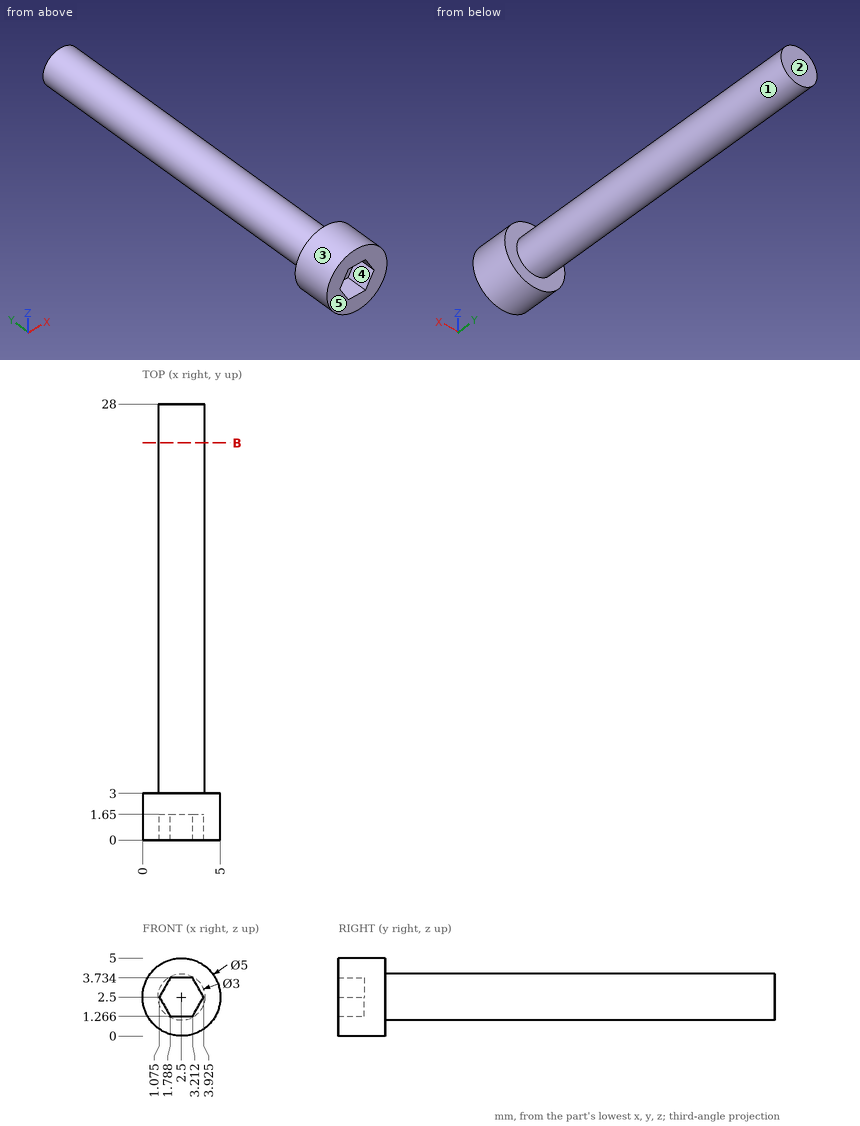
Job drawing, mm, ordinate dimensions from the low corner. One solid piece. A direction names the side the tool comes from. Coordinates: 2 decimals unless noted, no trailing zeros. Order: outer loops, then holes, each group sorted by start corner. A loop starts at its lowest first (then second) coordinate and runs counter-clockwise, first axis right, second up. Notation, with made-up numbers: (-7.75, 27) - (0.25, 27) arc R8 ccw to (0.25, 41) - close; hole circle Ø3 at (57.25, 27). An arc over 180 degrees is marked (long way). Return JSON: item names as keys, results as strings. Group by question number.
1) Flat gauge pin, fed straight in: P1, Ø1.5, axis at y = 12, z = 4, coming from the +X side. Where does the tip first touch, or does it go through?
2) Saw through at B-B, the plane y = 25.5. Write the cut outline in (x, z).
3) Probe line 1 (Y direction, x = 3.3, z = 2.35); line 2 (Y direction, x = 4, z = 3); line 3 (Z direction, x = 2.95, y = 23). List the from-to ranges inside material, lowest first. Write a range as from..to.
4) Mould opens along Z. For the marked faces 3, 4 and 5 say: released by +Z, released by -Z, zero draft, split by the parting line, or undercut.
5) Tool access for the marked faces 1 and 2: list every direction of +Z, -Z, +X, -X, +Y, -Y with a clear straight run to the whole face (end or side of a thin tool).
Values found:
{
 "1": {"P1": "stops at x = 3.8"},
 "2": {"outline": "circle Ø3 at (2.5, 2.5)"},
 "3": {"line 1": "y = 1.65..28", "line 2": "y = 0..3", "line 3": "z = 1.07..3.93"},
 "4": {"face 3": "split by the parting line", "face 4": "undercut", "face 5": "zero draft"},
 "5": {"face 1": "+Y", "face 2": "+Z, -Z, +X, -X, +Y"}
}
